from build123d import *

# Parameters (mm, degrees)
BOSS_EXTRUDE1_DEPTH = 2
SKETCH4_R           = 2
CUT_EXTRUDE1_DEPTH  = 10


with BuildPart() as part:
    # Sketch1 → Boss-Extrude1 (new body, symmetric)
    with BuildSketch(Plane.XY):
        Polygon((0, -5.773502692), (5, -2.886751346), (5, 2.886751346), (0, 5.773502692), (-5, 2.886751346), (-5, -2.886751346), align=None)
    extrude(amount=BOSS_EXTRUDE1_DEPTH, both=True)

    # Sketch3 → Cut-Revolve2 (revolve, cut)
    with BuildSketch(Plane(origin=(0, 0, 0), x_dir=(0, 0, -1), z_dir=(1, 0, 0))):
        with BuildLine():
            Line((-2, 4.773502692), (-3.338978682, 5.429088281))
            Line((-3.338978682, 5.429088281), (-2.142437664, 6.332858624))
            Line((-2.142437664, 6.332858624), (-1, 5.773502692))
            ThreePointArc((-1, 5.773502692), (-1.707106781, 5.480609473), (-2, 4.773502692))
        make_face()
    revolve(axis=Axis((0, 0, 0), (0, 0, 1)), mode=Mode.SUBTRACT)

    # Sketch4 → Cut-Extrude1 (cut)
    with BuildSketch(Plane.XY.offset(2)):
        Circle(SKETCH4_R)
    extrude(amount=-CUT_EXTRUDE1_DEPTH, mode=Mode.SUBTRACT)


solid = part.part
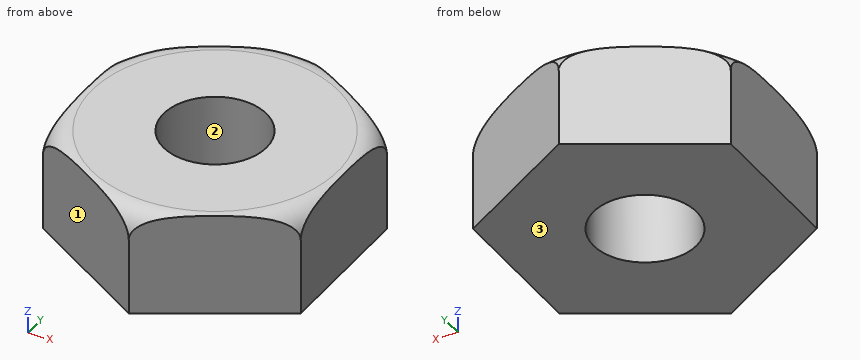
Here's how the part is built. I have some questions about the finished solid (model axes, mm). Face numbers are marked on the shaded views. Coordinates: 2 decimals unless noted, no trailing zeros. Loops run counter-clockwise (first coordinate to the right, second up) from the corner with the lowest first, then second, coordinate; pieces in that order, holes last. Notation, with made-up numbers: (25, 33.5) -> (68, 33.5) arc R25 ccw to (68, 59.5) -> close; hole circle Ø10 at (68.25, 4.25). An arc over 180 degrees is marked (long way). Use one line per item in the form item = value. Start each with the question number.
(1) Please list where these lines run through material, in increasing order: line 1 along Y through (x, z) = (1.75, 0.2); line 2 along X through (y, z) = (3.25, -0.1); line 3 along Y through (x, z) = (-4.5, -1.2).
(2) If we section it at A-A (y = 0): Please give me the cut outline in (x, z).
(3) We'd pull the mould along Y, two halves only. Please class the marked faces 1, 2 and 3: pulls with the +Y half, pulls with the -Y half, needs draft (parallel to the pull), parting line crosses it, or undercut.
(4) Will this pin go through, and if not, where does the flat tip stop? pin 1 (5 mm diameter, centred on x = 0, y = 0, fed in from -Z).
(5) If we section it at B-B (z = 0.2): Please give me the cut outline in (x, y), then the cut area to 3 significant figures.
Verdict:
q1.line_1 = -4.76 to -0.97, 0.97 to 4.76
q1.line_2 = -4.37 to 4.37
q1.line_3 = -3.18 to 3.18
q2.outline = (-5, -2) -> (-2, -2) -> (-2, 2) -> (-4.77, 2) arc R1 ccw to (-5, 1.97) -> close; (2, -2) -> (5, -2) -> (5, 1.97) arc R1 ccw to (4.77, 2) -> (2, 2) -> close
q3.face_1 = pulls with the -Y half
q3.face_2 = undercut
q3.face_3 = needs draft
q4.pin_1 = -2
q5.outline = (-5, -2.89) -> (0, -5.77) -> (5, -2.89) -> (5, 2.89) -> (0, 5.77) -> (-5, 2.89) -> close; hole circle Ø4 at (0, 0)
q5.area = 74.0 mm²
